Design review of the part built by this model. Coordinates are the model's own, in mm. A direction names the side the tool comes from. Coordinates: 2 decimals unless noted, no trailing zeros. Write each loop counter-clockwise with the first axis right and the second up, starting at its lowest first coordinate (ties: lowest second). Pieces come first, ordered by that corner, then holes. Notation, with made-up numbers: (42.5, -39.5) - (46.5, -39.5) arc R15 ccw to (46.5, -17.5) - close; hole circle Ø6 at (-35, -23.75). An arc over 180 degrees is marked (long way). One line per item, written item: value.
from build123d import *

# Parameters (mm, degrees)
SKETCH1_R           = 3.5
SKETCH1_R_2         = 0.6
BOSS_EXTRUDE1_DEPTH = 3


with BuildPart() as part:
    # Sketch1 → Boss-Extrude1 (new body)
    with BuildSketch(Plane.XY):
        with BuildLine():
            ThreePointArc((2.256436303, 18.02221908), (1.945672304, 19.349065897), (1.067466411, 20.391107713))
            ThreePointArc((1.067466411, 20.391107713), (0.855450056, 20.341742586), (0.644777778, 20.286924322))
            ThreePointArc((0.644777778, 20.286924322), (0.351426057, 18.956119489), (0.692874662, 17.636835748))
            ThreePointArc((0.692874662, 17.636835748), (0.130369461, 17.378260197), (-0.40197342, 17.062215148))
            ThreePointArc((-0.40197342, 17.062215148), (-1.293757737, 18.092660425), (-2.555631415, 18.607220002))
            ThreePointArc((-2.555631415, 18.607220002), (-2.720421456, 18.464980439), (-2.881487176, 18.318536988))
            ThreePointArc((-2.881487176, 18.318536988), (-2.522781382, 17.003840487), (-1.607341932, 15.994351828))
            ThreePointArc((-1.607341932, 15.994351828), (-1.985249501, 15.503985347), (-2.309742255, 14.976749281))
            ThreePointArc((-2.309742255, 14.976749281), (-3.57824985, 15.474730425), (-4.93471126, 15.343928364))
            ThreePointArc((-4.93471126, 15.343928364), (-5.014523575, 15.141399736), (-5.089084522, 14.936879527))
            ThreePointArc((-5.089084522, 14.936879527), (-4.160496386, 13.939472483), (-2.880782238, 13.471040593))
            ThreePointArc((-2.880782238, 13.471040593), (-2.987518106, 12.861220233), (-3.029823353, 12.243576579))
            ThreePointArc((-3.029823353, 12.243576579), (-4.384454423, 12.09501211), (-5.524754604, 11.348813588))
            ThreePointArc((-5.524754604, 11.348813588), (-5.501305152, 11.132392762), (-5.472280312, 10.916648911))
            ThreePointArc((-5.472280312, 10.916648911), (-4.186538186, 10.465025257), (-2.835716429, 10.644962236))
            ThreePointArc((-2.835716429, 10.644962236), (-2.646828694, 10.055390493), (-2.397254812, 9.488833969))
            ThreePointArc((-2.397254812, 9.488833969), (-3.527679704, 8.727758217), (-4.190589627, 7.537108322))
            ThreePointArc((-4.190589627, 7.537108322), (-4.069250395, 7.356374701), (-3.943289009, 7.178831524))
            ThreePointArc((-3.943289009, 7.178831524), (-2.594940919, 7.376452797), (-1.482468538, 8.163537251))
            ThreePointArc((-1.482468538, 8.163537251), (-1.041229104, 7.729277906), (-0.556950462, 7.343599785))
            ThreePointArc((-0.556950462, 7.343599785), (-1.204202457, 6.144366032), (-1.237857446, 4.782028306))
            ThreePointArc((-1.237857446, 4.782028306), (-1.046425791, 4.678385785), (-0.852384094, 4.579716284))
            ThreePointArc((-0.852384094, 4.579716284), (0.249679662, 5.381309833), (0.868948651, 6.595230199))
            ThreePointArc((0.868948651, 6.595230199), (1.461457147, 6.415766834), (2.069498148, 6.299321325))
            ThreePointArc((2.069498148, 6.299321325), (2.053696683, 4.936659572), (2.657006579, 3.714729171))
            ThreePointArc((2.657006579, 3.714729171), (2.874675973, 3.711921002), (3.092345367, 3.714729171))
            ThreePointArc((3.092345367, 3.714729171), (3.695655263, 4.936659572), (3.679853798, 6.299321325))
            ThreePointArc((3.679853798, 6.299321325), (4.2878948, 6.415766834), (4.880403295, 6.595230199))
            ThreePointArc((4.880403295, 6.595230199), (5.499672285, 5.381309833), (6.60173604, 4.579716284))
            ThreePointArc((6.60173604, 4.579716284), (6.795777737, 4.678385785), (6.987209392, 4.782028306))
            ThreePointArc((6.987209392, 4.782028306), (6.953554403, 6.144366032), (6.306302409, 7.343599785))
            ThreePointArc((6.306302409, 7.343599785), (6.790581051, 7.729277906), (7.231820484, 8.163537251))
            ThreePointArc((7.231820484, 8.163537251), (8.344292866, 7.376452797), (9.692640955, 7.178831524))
            ThreePointArc((9.692640955, 7.178831524), (9.818602342, 7.356374701), (9.939941573, 7.537108322))
            ThreePointArc((9.939941573, 7.537108322), (9.27703165, 8.727758217), (8.146606758, 9.488833969))
            ThreePointArc((8.146606758, 9.488833969), (8.39618064, 10.055390493), (8.585068375, 10.644962236))
            ThreePointArc((8.585068375, 10.644962236), (9.935890133, 10.465025257), (11.221632258, 10.916648911))
            ThreePointArc((11.221632258, 10.916648911), (11.250657098, 11.132392762), (11.27410655, 11.348813588))
            ThreePointArc((11.27410655, 11.348813588), (10.133806369, 12.09501211), (8.779175299, 12.243576579))
            ThreePointArc((8.779175299, 12.243576579), (8.736870052, 12.861220233), (8.630134184, 13.471040593))
            ThreePointArc((8.630134184, 13.471040593), (9.909848333, 13.939472483), (10.838436468, 14.936879527))
            ThreePointArc((10.838436468, 14.936879527), (10.763875521, 15.141399736), (10.684063206, 15.343928364))
            ThreePointArc((10.684063206, 15.343928364), (9.327601796, 15.474730425), (8.059094201, 14.976749281))
            ThreePointArc((8.059094201, 14.976749281), (7.734601447, 15.503985347), (7.356693878, 15.994351828))
            ThreePointArc((7.356693878, 15.994351828), (8.272133328, 17.003840487), (8.630839122, 18.318536988))
            ThreePointArc((8.630839122, 18.318536988), (8.469773402, 18.464980439), (8.304983361, 18.607220002))
            ThreePointArc((8.304983361, 18.607220002), (7.043109683, 18.092660425), (6.151325366, 17.062215148))
            ThreePointArc((6.151325366, 17.062215148), (5.618982485, 17.378260197), (5.056477284, 17.636835748))
            ThreePointArc((5.056477284, 17.636835748), (5.39792589, 18.956119489), (5.104574168, 20.286924322))
            ThreePointArc((5.104574168, 20.286924322), (4.893901891, 20.341742586), (4.681885535, 20.391107713))
            ThreePointArc((4.681885535, 20.391107713), (3.803679642, 19.349065897), (3.492915643, 18.02221908))
            ThreePointArc((3.492915643, 18.02221908), (2.874675973, 18.054671002), (2.256436303, 18.02221908))
        make_face()
        with Locations((2.874675973, 12.149421002)):
            Circle(SKETCH1_R, mode=Mode.SUBTRACT)
        with Locations((-0.135327396, 15.426977975)):
            Circle(SKETCH1_R_2, mode=Mode.SUBTRACT)
    extrude(amount=BOSS_EXTRUDE1_DEPTH)


solid = part.part
1. Consider section C-C, the plane z = 0.25. Give the number of separate pieces and of enclosed holes in the cut face, then the cut area to 3 significant figures.
Answer block:
separate pieces: 1
enclosed holes: 2
area: 118 mm^2
2. Consider section B-B, the plane y = 10.25. Write out the cut boundary in (x, z), then the cut area to 3 significant figures.
Answer block:
outline: (-2.72, 0) - (-0.07, 0) - (-0.07, 3) - (-2.72, 3) - close; (5.81, 0) - (8.47, 0) - (8.47, 3) - (5.81, 3) - close
area: 15.9 mm^2
3. Mouldability with a two-part tool opening along Y and no side actions: class faces 4 (the face through (9.917, 10.463, 1.479)), 5 (the face through (3, 8, 0)), 6 (the face through (-4.37, 12.1, 1.48)) as released by +Y, released by -Y, zero draft, split by the parting line, or undercut.
Answer block:
face 4: undercut
face 5: zero draft
face 6: undercut
4. Wall thickness on line 1 along Y through (x, z) = (-3.25, 0.2); line 2 along Y through (x, z) = (0.25, 2.3); line 3 along X through (y, z) = (17.75, 2.1): over which ranges is each line inside the solid? List them lowest first.
Answer block:
line 1: y = 7.2 to 8.99, 10.52 to 12.26, 13.54 to 15.41
line 2: y = 5.38 to 9.83, 14.46 to 14.97, 15.89 to 17.44
line 3: x = -2.81 to -0.9, 0.64 to 5.11, 6.65 to 8.56
5. Insertion check: pin 1 Ø1.1 at (x, y) = (-0.14, 15.43) entering from +Z; pin 2 Ø1 at (x, z) = (9.5, 2.5) entering from +Y; pin 3 Ø1 at (y, z) = (14, 2.5) entering from -X. Each pin has a flat end and moves straight along its axis. Give the tip position at first contact, or say it passes through.
Answer block:
pin 1: passes through
pin 2: stops at y = 15.5
pin 3: stops at x = -4.79
6. For faces 1 (the face through (-1.98, 15.51, 1.48)), 2 (the face through (-4.177, 13.95, 1.479)), 3 (the face through (3, 8, 3)), list the 3-axis set-ups (+Z, -Z, +X, -X, +Y, -Y) from which the entire face can be reached by the end or side of a thin tool; tool diameter is ignored.
Answer block:
face 1: +Z, -Z
face 2: +Z, -Z, -X
face 3: +Z, +X, -X, +Y, -Y
7. Consider section A-A, the plane y = 14.5. Write out the cut boundary in (x, z).
Answer block:
outline: (-4.79, 0) - (0.28, 0) - (0.28, 3) - (-4.79, 3) - close; (5.47, 0) - (10.54, 0) - (10.54, 3) - (5.47, 3) - close
